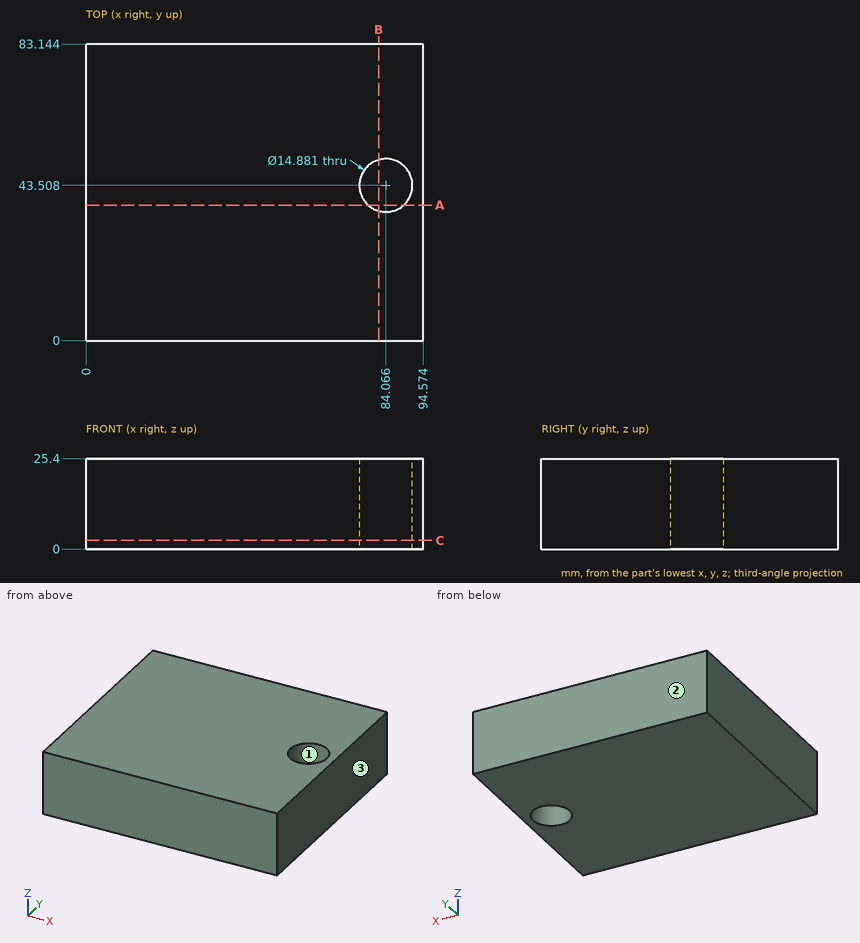
Check sheet for the drawn part. Datum: minimum x, y, z corner. Units: mm. Give positions to 0.01 mm unless a question says otherwise; leave off trailing zeros. Write each loop counter-clockwise with the first axis right and the second up, starting at its lowest first coordinate (ties: lowest second). Pieces come first, ordered by that corner, then holes. Notation, with made-up numbers: (13.25, 19) -> (51.25, 19) arc R11 cw to (51.25, 28) -> close; hole circle Ø4 at (15.25, -25). An arc over 180 degrees is marked (long way). Use one line per item in the form item = value. Start each with the question number.
1. Section check A-A (y = 38). Record the cut outline in (x, z).
2. Mould release check, pull along Y, two halves, no side actions. Record for the marked faces 1, 2 and 3: pulls with the +Y half, pulls with the -Y half, needs draft (parallel to the pull), parting line crosses it, or undercut.
3. Thickness scan on line 1 along Y through (x, z) = (80, 14.75) (1 decimal); line 2 along Y through (x, z) = (89.5, 8.25) (1 decimal). Record the ranges inside material, lowest first. Write a range as from..to.
4. Section check B-B (x = 82). Record the cut outline in (y, z).
5. Section check C-C (z = 2.5). Record the cut outline in (x, y) (1 decimal), and give its area (3 significant figures).
Conclusion:
q1.outline = (0, 0) -> (79.06, 0) -> (79.06, 25.4) -> (0, 25.4) -> close; (89.07, 0) -> (94.57, 0) -> (94.57, 25.4) -> (89.07, 25.4) -> close
q2.face_1 = undercut
q2.face_2 = pulls with the +Y half
q2.face_3 = needs draft
q3.line_1 = 0..37.3, 49.7..83.1
q3.line_2 = 0..38.4, 48.6..83.1
q4.outline = (0, 0) -> (36.36, 0) -> (36.36, 25.4) -> (0, 25.4) -> close; (50.66, 0) -> (83.14, 0) -> (83.14, 25.4) -> (50.66, 25.4) -> close
q5.outline = (0, 0) -> (94.6, 0) -> (94.6, 83.1) -> (0, 83.1) -> close; hole circle Ø14.9 at (84.1, 43.5)
q5.area = 7,690 mm²
